Geometry check sheet. Reference: the model listing, model coordinates, mm. Face numbers are marked on the shaded views. A direction names the side the tool comes from. Round coordinates to 2 decimals unless told otherwise and drop trailing zeros. Loops run counter-clockwise (first coordinate to the right, second up) from the corner with the lowest first, then second, coordinate; pieces in that order, holes last. Notation, with made-up numbers: (35, -16.75) - (74, -16.75) arc R20 cw to (74, 8.25) - close; hole circle Ø10 at (-23.5, 79). An arc over 180 degrees is marked (long way). Answer in a Markdown table with one row per item. Add a question column.
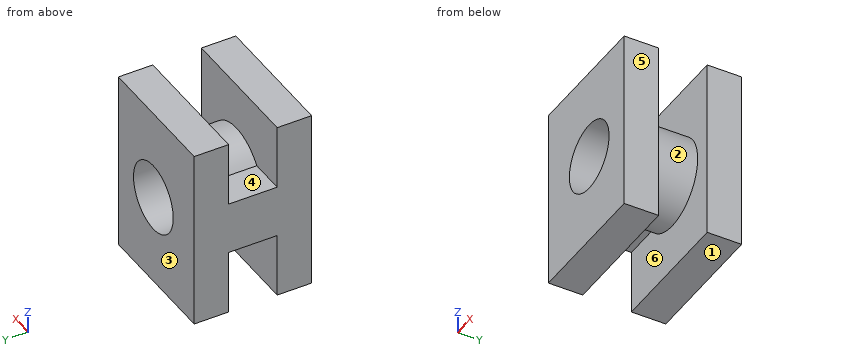
Autodesk Inventor part; units mm, degrees
ref_plane "YZ Plane" through (0, 0, 0) normal (1, 0, 0) x (0, 1, 0)
ref_plane "XZ Plane" through (0, 0, 0) normal (0, 1, 0) x (-1, 0, 0)
ref_plane "XY Plane" through (0, 0, 0) normal (0, 0, 1) x (1, 0, 0)
sketch "Sketch1" plane through (0, 0, 0) normal (0, 1, 0) x (-1, 0, 0)
  line L0 (0, 0) -> (6.5, 0)
  line L1 (6.5, 0) -> (6.5, -9)
  line L2 (6.5, -9) -> (0, -9)
  line L3 (0, 0) -> (0, -9)
  dimension "d0" = 6.5
  dimension "d1" = 9
extrude "Extrusion1" add sketch "Sketch1" along normal blind 1.7
sketch "Sketch2" plane through (0, 1.7, 0) normal (0, 1, 0) x (1, 0, 0)
  circle A0 centre (-3, 4.5) radius 1.7
  dimension "d9" = 3.4
extrude "Extrusion2" cut sketch "Sketch2" against normal blind 1.7
sketch "Sketch3" plane through (0, 1.7, 0) normal (0, 1, 0) x (1, 0, 0)
  circle A0 centre (-3, 4.5) radius 2.18
  line L0 (-6.5, 3.2) -> (-4.75, 3.2)
  line L1 (-6.5, 5.8) -> (-4.75, 5.8)
  line L2 (-6.5, 3.2) -> (-6.5, 5.8)
  line L3 (-6.5, 9) -> (-6.5, 0)
  dimension "d12" = 4.36
extrude "Extrusion3" add sketch "Sketch3" along normal blind 2.4
sketch "Sketch4" plane through (0, 4.1, 0) normal (0, 1, 0) x (1, 0, 0)
  line L0 (-6.5, 0) -> (0, 0)
  line L1 (-6.5, 9) -> (-6.5, 5.8)
  line L2 (0, 0) -> (-6.5, 0)
  line L3 (-6.5, 0) -> (-6.5, 9)
  line L4 (-6.5, 9) -> (0, 9)
  line L5 (0, 9) -> (0, 0)
extrude "Extrusion4" add sketch "Sketch4" along normal blind 1.7
sketch "Sketch5" plane through (0, 5.8, 0) normal (0, 1, 0) x (1, 0, 0)
  circle A0 centre (-3, 4.5) radius 1.7
  circle A1 centre (-3, 4.5) radius 1.7
  dimension "d20" = 3.4
extrude "Extrusion5" cut sketch "Sketch5" against normal blind 5.8
properties part number "MMAE 232 Assignment 2_Rubber Grommet - Dylan Tamras"
Q1. Scan lines: line 1 (Y direction, x = -1.75, z = -0.5); line 2 (Z direction, x = -3, y = 1.75); line 3 (X direction, y = 3.1, z = -4.5). Record each from-to range of solid material in increasing order. Write a range as from..to.
Q2. Release check for a two-part mould opening along Y. For the marked faces 1, 2 and 3 record: +Y half, -Y half, draft (parallel to the pull), parting line (faces both ways), or undercut.
Q3. Cross-section at B-B, the plane x = -3. Enter the section's corners in (y, z), plus the area to 3 significant figures.
Q4. Set-up check for the marked faces 4, 5 and 6: record each of +Z, -Z, +X, -X, +Y, -Y from which the full face is reachable in a straight line by a thin tool's end or side.
Q5. Cross-section at A-A, the plane z = -4.5. Enter the section's corners in (x, y), plus the area to 3 significant figures.
Q6. Cross-section at C-C, the plane z = -7. Enter the section's corners in (x, y), plus the area to 3 significant figures.
Q7. Depth check by flat-ended pin: P1, Ø2, axis at x = -4.5, y = 3.5, coming from the -Z side; P2, Ø1.5, axis at x = -2, y = 2.5, coming from the -Z side; P3, Ø2.5, axis at x = -3, z = -4.5, coming from the -Y side; P4, Ø1.4, axis at x = -5.5, y = 3, coming from the +Z side. Enter the tip coordinate at first touch or a pass-through.
Q8. Cross-section at D-D, the plane y = 0.7. Enter the section's corners in (x, z), plus the area to 3 significant figures.
Check sheet entries:
| question | item | result |
|---|---|---|
| 1 | line 1 | 0..1.7, 4.1..5.8 |
| 1 | line 2 | -6.68..-6.2, -2.8..-2.32 |
| 1 | line 3 | -6.5..-4.7, -1.3..-0.82 |
| 2 | face 1 | draft |
| 2 | face 2 | undercut |
| 2 | face 3 | +Y half |
| 3 | outline | (0, -9) - (1.7, -9) - (1.7, -6.68) - (4.1, -6.68) - (4.1, -9) - (5.8, -9) - (5.8, -6.2) - (0, -6.2) - close; (0, -2.8) - (5.8, -2.8) - (5.8, 0) - (4.1, 0) - (4.1, -2.32) - (1.7, -2.32) - (1.7, 0) - (0, 0) - close |
| 3 | area | 21.3 mm² |
| 4 | face 4 | +Z, -X |
| 4 | face 5 | +Z, -Z, +X, +Y, -Y |
| 4 | face 6 | none |
| 5 | outline | (-6.5, 0) - (-4.7, 0) - (-4.7, 5.8) - (-6.5, 5.8) - close; (-1.3, 0) - (0, 0) - (0, 1.7) - (-0.82, 1.7) - (-0.82, 4.1) - (0, 4.1) - (0, 5.8) - (-1.3, 5.8) - close |
| 5 | area | 16.0 mm² |
| 6 | outline | (-6.5, 0) - (0, 0) - (0, 1.7) - (-6.5, 1.7) - close; (-6.5, 4.1) - (0, 4.1) - (0, 5.8) - (-6.5, 5.8) - close |
| 6 | area | 22.1 mm² |
| 7 | P1 | z = -9 |
| 7 | P2 | z = -6.67 |
| 7 | P3 | through |
| 7 | P4 | z = -3.2 |
| 8 | outline | (-6.5, -9) - (0, -9) - (0, 0) - (-6.5, 0) - close; hole circle Ø3.4 at (-3, -4.5) |
| 8 | area | 49.4 mm² |
